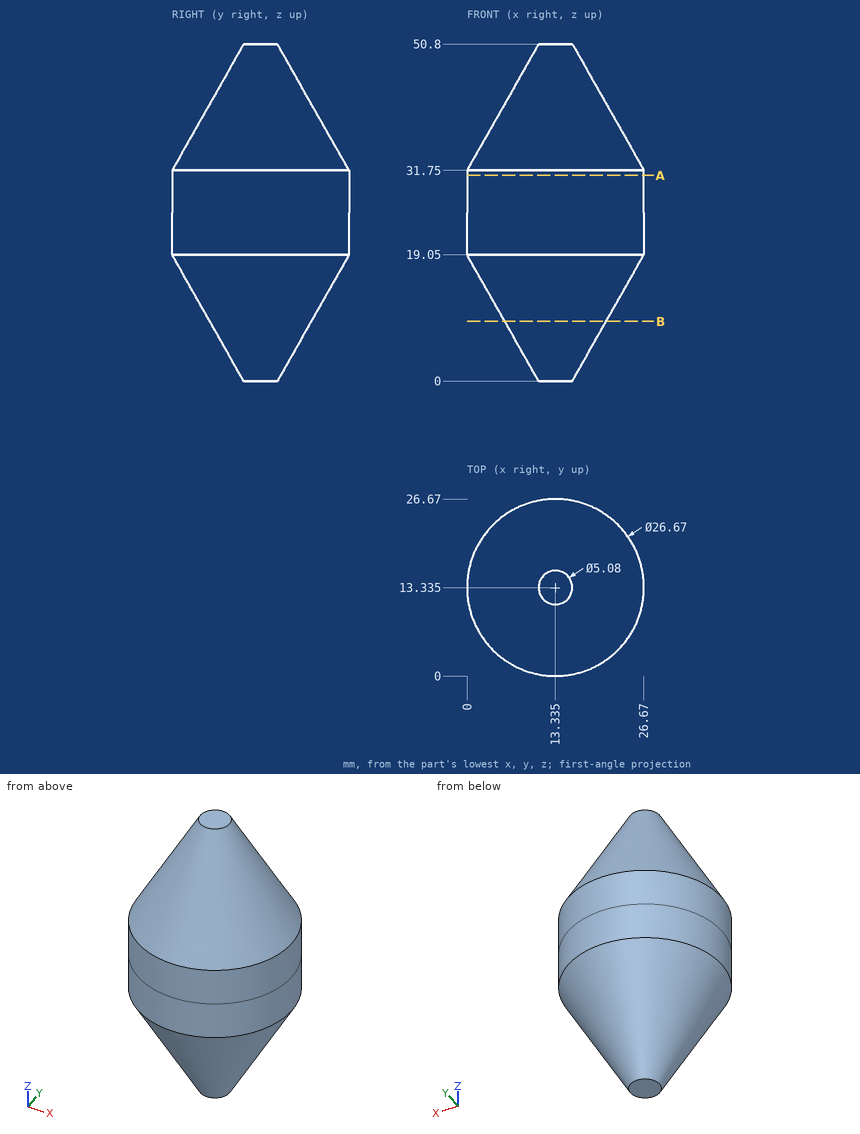
Answer from the drawing. Dimensions are ordinates in mm from the lowest x, y and z of the part. Coordinates: 2 decimals unless noted, no trailing zeros. Write each loop counter-clockwise with the first axis right and the second up, starting at its lowest first coordinate (ties: lowest second). Pieces come first, ordered by that corner, then holes. Notation, with made-up numbers: (11, 0.25) - (51, 0.25) arc R35 ccw to (51, 33.25) - close; hole circle Ø4 at (14.5, 15). An arc over 180 degrees is marked (long way). Return JSON: item names as keys, results as strings. Group by question number.
Q1. The part is cut by section B-B on z = 9. Write down the section's boundary in (x, y) (3 decimals).
Q2. Flat-ended cylindrical pins translate along their axes: pin 1 Ø4 at (x, y) = (20.5, 15) entering from -Z; pin 2 Ø1 at (x, z) = (8.5, 34) entering from -Y; pin 3 Ø1 at (y, z) = (13, 29.5) entering from +X; pin 4 Ø1 at (y, z) = (13.5, 13.5) entering from -X. Find the tip coordinate at first contact, or state that the pin passes through.
Q3. The part is cut by section A-A on z = 31. Write down the section's boundary in (x, y) (3 decimals), and give its area (3 significant figures).
Q4. Find the intervals of material crossed by line 1 along Y through (x, z) = (4.5, 24.5); line 2 along Z through (x, y) = (8, 18.25); line 3 along Z through (x, y) = (20, 2), in increasing order. Write a range as [from, to].
Evaluation:
{
 "1": {"outline": "circle Ø15.28 at (13.335, 13.335)"},
 "2": {"pin 1": "stops at z = 4.97", "pin 2": "stops at y = 1.92", "pin 3": "stops at x = 26.67", "pin 4": "stops at x = 2.86"},
 "3": {"outline": "circle Ø26.67 at (13.335, 13.335)", "area": "559 mm2"},
 "4": {"line 1": "y = [3.35, 23.32]", "line 2": "z = [8.32, 42.48]", "line 3": "z = [18.72, 32.08]"}
}
